Part model, mm, in its own coordinate system. Face numbers are marked on the shaded views. A direction names the side the tool comes from. Give positions to 0.01 mm unless a question says otherwise; leave off trailing zeros. Loops run counter-clockwise (first coordinate to the right, second up) from the corner with the lowest first, then second, coordinate; pieces in that order, holes last. Notation, with made-up numbers: M 75,37.5 L 96,37.5 A4 cw 96,43.5 Z; hole C 80,-11 d1. An arc over 180 degrees is marked long. Answer in a Markdown table with one row per item.
from build123d import *

# Parameters (mm, degrees)
SKETCH1_R           = 1.5
BOSS_EXTRUDE1_DEPTH = 2
BOSS_EXTRUDE2_START = -2
SKETCH2_R           = 0.514521653
BOSS_EXTRUDE2_DEPTH = 2


with BuildPart() as part:
    # Sketch1 → Boss-Extrude1 (new body)
    with BuildSketch(Plane(origin=(0, 0, 0), x_dir=(1, 0, 0), z_dir=(0, 1, 0))):
        with BuildLine():
            Line((2.247922133, -3.308601832), (8.796170176, -2.191071372))
            ThreePointArc((8.796170176, -2.191071372), (12.441065174, -0.53963026), (9.831944444, 2.49434507))
            ThreePointArc((9.831944444, 2.49434507), (5.556167823, 2.665089568), (1.414583333, 3.741517606))
            ThreePointArc((1.414583333, 3.741517606), (-3.972345981, -0.469539568), (2.247922133, -3.308601832))
        make_face()
        with Locations(Location((0, 0, 0), (0, 0, 270))):
            Circle(SKETCH1_R, mode=Mode.SUBTRACT)
    extrude(amount=BOSS_EXTRUDE1_DEPTH)

    # Sketch2 → Boss-Extrude2 (add)
    with BuildSketch(Plane(origin=(0, 2, 0), x_dir=(1, 0, 0), z_dir=(0, 1, 0)).offset(BOSS_EXTRUDE2_START)):
        with BuildLine():
            Line((-5.984144072, 4.635311674), (0.408466301, 3.979089755))
            ThreePointArc((0.408466301, 3.979089755), (-3.466544022, 1.995763648), (-3.236020649, -2.35120615))
            Line((-3.236020649, -2.35120615), (-7.013353091, 2.847625854))
            ThreePointArc((-7.013353091, 2.847625854), (-7.078453265, 4.075217168), (-5.984144072, 4.635311674))
        make_face()
        with Locations(Location((-6.099495617, 3.51161028, 0), (0, 0, 270))):
            Circle(SKETCH2_R, mode=Mode.SUBTRACT)
    extrude(amount=BOSS_EXTRUDE2_DEPTH)


solid = part.part
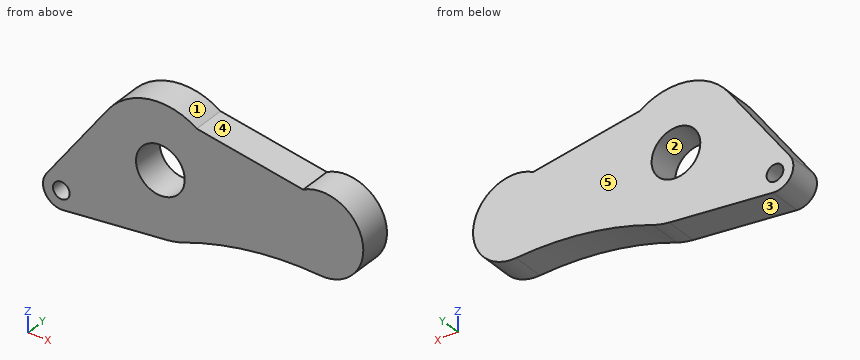
(1) Which spindle directions (+Z, -Z, +X, -X, +Y, -Y) get a long thin tool onto all of the face, cutting with end or side? Do the marked faces 4 and 5. Say none if no direction does.
Recorded:
| item | result |
|---|---|
| face 4 | +Z, +Y, -Y |
| face 5 | +Z, -Z, +X, -X, +Y |
(2) Saw through at A-A (y = 1.4). Write the cut outline in (x, z), plus the area to 3 significant figures.
Recorded:
| item | result |
|---|---|
| outline | M -7.01,-2.85 A1.13 ccw -5.98,-4.64 L 0.41,-3.98 A4 ccw 1.41,-3.74 A20 cw 9.83,-2.49 A2.5 ccw long 8.8,2.19 L 2.25,3.31 A4 ccw -3.24,2.35 Z; hole C -6.1,-3.51 d1.03; hole C 0,0 d3 |
| area | 102 mm^2 |
(3) Pull direction X, two halves, no side cores. Call the marked faces 1, 2 and 3: +X half, -X half, draft (parallel to the pull), parting line (faces both ways), or undercut.
Recorded:
| item | result |
|---|---|
| face 1 | parting line |
| face 2 | undercut |
| face 3 | +X half |
(4) Saw through at D-D (x = 11.25). Write the cut outline in (y, z).
Recorded:
| item | result |
|---|---|
| outline | M 0,-2.17 L 2,-2.17 L 2,2.17 L 0,2.17 Z |
(5) Saw through at C-C (x = 0). Write the cut outline in (y, z).
Recorded:
| item | result |
|---|---|
| outline | M 0,-4.02 L 2,-4.02 L 2,-1.5 L 0,-1.5 Z; M 0,1.5 L 2,1.5 L 2,4 L 0,4 Z |
(6) Saw through at B-B (z = 0). Write the cut outline in (x, y), plus the area to 3 significant figures.
Recorded:
| item | result |
|---|---|
| outline | M -4.94,0 L -1.5,0 L -1.5,2 L -4.94,2 Z; M 1.5,0 L 12.5,0 L 12.5,2 L 1.5,2 Z |
| area | 28.9 mm^2 |
(7) Pin check, flat tip, straight feed: pin 1 Ø1.8 at (x, z) = (0, 0) entering from -Y. Stop position of the tip, or through.
Recorded:
| item | result |
|---|---|
| pin 1 | passes through |
(8) Drill centre lines: line 1 along X through (y, z) = (1.1, -1.25); line 2 along X through (y, z) = (0.8, 0); line 3 along Z through (x, y) = (-1, 1.3). Where is each one in solid material? Low to high.
Recorded:
| item | result |
|---|---|
| line 1 | x = -5.85 to -0.83, 0.83 to 12.17 |
| line 2 | x = -4.94 to -1.5, 1.5 to 12.5 |
| line 3 | z = -4.12 to -1.12, 1.12 to 3.87 |
